Geometry: final body of the model. Coordinates: model frame, mm. A direction names the side the tool comes from. Round coordinates to 2 decimals unless told otherwise and drop trailing zeros. Loops run counter-clockwise (first coordinate to the right, second up) from the corner with the lowest first, then second, coordinate; pieces in that order, holes last. Notation, with made-up numbers: (13.5, -31.75) - (56.5, -31.75) arc R18 ccw to (56.5, -20.75) - close; hole circle Ø5 at (74.5, 48.5). An arc over 180 degrees is marked (long way). Return JSON: item names as keys, results as strings. Group by question number.
1. Material intervals for probe 1 along Z at (x, y) = (-1.2, 8.75); probe 2 along X at (y, z) = (3.25, -0.05); probe 3 along X at (y, z) = (8.5, -0.55), sorted ascending.
2. First-contact query: pin 1 Ø0.7 at (y, z) = (9, 1) entering from -X; pin 2 Ø1 at (x, z) = (-1.5, 1) entering from +Y; pin 3 Ø3 at (x, y) = (0, 2) entering from +Z. Flat tips, straight axial feed; report the tip coordinate or a pass-through.
3. Draft query along X for faces 3 (the face through (-1, 9, 0.381)), 4 (the face through (-0.17, 3.86, -1.26)), 5 (the face through (1.3, 7.62, 0.6)). Return one class per face: +X half, -X half, draft (parallel to the pull), parting line (faces both ways), or undercut.
4. Set-up query: faces 1 (the face through (0.381, 9, -1)), 2 (the face through (0, 0, 0)). Return all of +Z, -Z, +X, -X, +Y, -Y with unobstructed straight access to the full face (end or side cutting, diameter ignored); none if empty.
5. Section A-A on y = 7.25. Return loops of the section in (x, z), and give its area (3 significant figures).
from build123d import *

# Parameters (mm, degrees)
REVOLVE1_OUTLINE_W = 1.27
REVOLVE1_OUTLINE_H = 7.62
SKETCH2_W          = 1.27
SKETCH2_H          = 0.762
CUT_EXTRUDE1_DEPTH = 1.27
CIRPATTERN1_COUNT  = 4


# Read off the part's stored shape, not the designer's step: Revolve1
with BuildPart() as part:
    # Revolve1 outline → Revolve1 (revolve)
    with BuildSketch(Plane.XY):
        with Locations((0.635, 3.81)):
            Rectangle(REVOLVE1_OUTLINE_W, REVOLVE1_OUTLINE_H)
        with BuildLine():
            Line((0, 9.525), (0, 7.62))
            Line((0, 7.62), (1.27, 7.62))
            Line((1.27, 7.62), (1.27, 9.421457579))
            add(Edge.make_bspline(
                [(1.27, 9.421457579), (1.228139819, 9.428026655), (0.811912502, 9.488262021), (0.384414806, 9.507605733), (0, 9.525)],
                knots=[0.678395856, 0.678395856, 0.678395856, 0.678395856, 0.710806875, 1, 1, 1, 1], degree=3))
        make_face()
        with BuildLine():
            Line((1.27, 9.421457579), (1.27, 7.62))
            Line((1.27, 7.62), (2.7305, 7.62))
            add(Edge.make_bspline(
                [(2.7305, 7.62), (2.730181564, 7.703312624), (2.729863127, 7.786625248), (2.7305, 7.873222802)],
                knots=[0, 0, 0, 0, 0.063828226, 0.063828226, 0.063828226, 0.063828226], degree=3))
            Line((2.7305, 7.873222802), (2.7305, 8.214607098))
            add(Edge.make_bspline(
                [(2.7305, 8.214607098), (2.72332571, 8.473946678), (2.657632203, 8.947113323), (1.963979921, 9.279802566), (1.518244272, 9.38250086), (1.27, 9.421457579)],
                knots=[0.145285385, 0.145285385, 0.145285385, 0.145285385, 0.328975575, 0.486188137, 0.678395856, 0.678395856, 0.678395856, 0.678395856], degree=3))
        make_face()
        with BuildLine():
            Line((2.7305, 8.214607098), (2.7305, 7.873222802))
            add(Edge.make_bspline(
                [(2.7305, 7.873222802), (2.731005418, 7.941946006), (2.73211248, 8.012738026), (2.73211248, 8.084105221)],
                knots=[0.063828226, 0.063828226, 0.063828226, 0.063828226, 0.114481853, 0.114481853, 0.114481853, 0.114481853], degree=3))
            add(Edge.make_bspline(
                [(2.73211248, 8.084105221), (2.73211248, 8.127505109), (2.731703077, 8.171117703), (2.7305, 8.214607098)],
                knots=[0.114481853, 0.114481853, 0.114481853, 0.114481853, 0.145285385, 0.145285385, 0.145285385, 0.145285385], degree=3))
        make_face()
    revolve(axis=Axis((0, 0, 0), (0, 1, 0)))

    # Sketch2 → Cut-Extrude1 (cut)
    with BuildSketch(Plane.XZ.offset(-9.525)):
        with Locations((0.635, 0)):
            Rectangle(SKETCH2_W, SKETCH2_H)
    cut_extrude1 = extrude(amount=CUT_EXTRUDE1_DEPTH, mode=Mode.SUBTRACT)

    # CirPattern1: Cut-Extrude1 ×4 about axis
    cirpattern1_axis = Axis((0, 0, 0), (0, 1, 0))
    for i in range(1, CIRPATTERN1_COUNT):
        add(cut_extrude1.rotate(cirpattern1_axis, i * 360 / CIRPATTERN1_COUNT), mode=Mode.SUBTRACT)


solid = part.part
Taken from the geometry:
{
 "1": {"probe 1": "-2.35 to -0.38, 0.38 to 2.35", "probe 2": "-1.27 to 1.27", "probe 3": "-2.65 to -0.38, 0.38 to 2.65"},
 "2": {"pin 1": "x = -2.53", "pin 2": "y = 9.42", "pin 3": "z = 1.27"},
 "3": {"face 3": "undercut", "face 4": "parting line", "face 5": "draft"},
 "4": {"face 1": "+Y", "face 2": "+Z, -Z, +X, -X, -Y"},
 "5": {"outline": "circle Ø2.54 at (0, 0)", "area": "5.07 mm2"}
}
